Source: three-view drawing plus pictorial views. Frame: mm from the lowest corner of the part. A direction names the side the tool comes from. Give positions to 0.01 mm unless a question says otherwise; leave off trailing zeros. Loops run counter-clockwise (first coordinate to the right, second up) from the corner with the lowest first, then second, coordinate; pieces in that order, holes last. Notation, with made-up numbers: (47, -34.75) -> (102, -34.75) arc R15 cw to (102, -17.75) -> close; hole circle Ø1 at (37.25, 72.25). An arc over 180 degrees is marked (long way). Put each result on its own line as item: value.
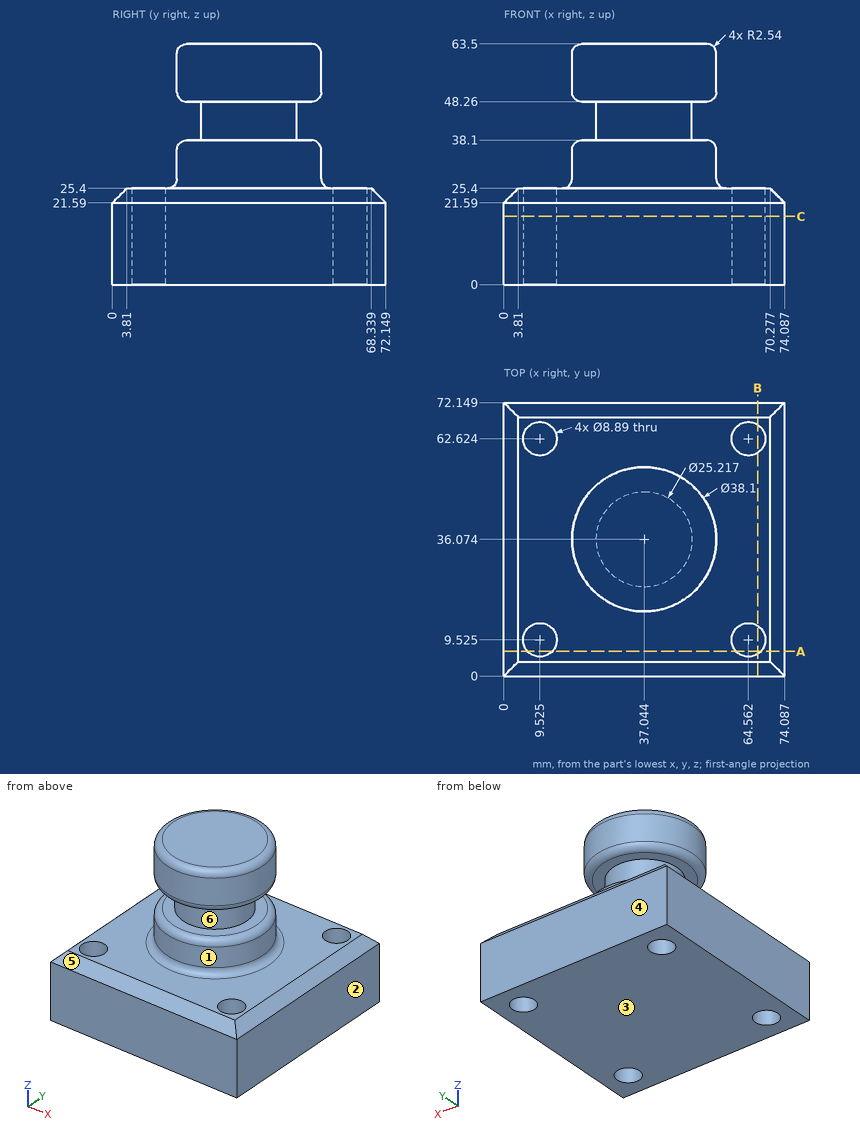
(1) First-contact query: P1, Ø4, axis at x = 31.5, z = 57, coming from the +Y side; P2, Ø12, axis at y = 16, z = 29, coming from the -X side; P3, Ø12, axis at x = 58.5, y = 14, coming from the +Z side. Flat tips, straight axial feed; report the tip coordinate or a pass-through.
Calculated:
P1: stops at y = 54.79
P2: stops at x = 1.41
P3: stops at z = 25.4
(2) Section A-A on y = 6.5. Return loops of the section in (x, z) (1 decimal).
Calculated:
outline: (0, 0) -> (6.3, 0) -> (6.3, 25.4) -> (3.8, 25.4) -> (0, 21.6) -> close; (12.8, 0) -> (61.3, 0) -> (61.3, 25.4) -> (12.8, 25.4) -> close; (67.8, 0) -> (74.1, 0) -> (74.1, 21.6) -> (70.3, 25.4) -> (67.8, 25.4) -> close
(3) Line query: probe 1 along Y at (x, z) = (10.5, 6); probe 2 along Z at (x, y) = (13, 4); probe 3 along Y at (x, z) = (9, 15). Output: solid intervals per line, ascending. Write a range as from..to.
Calculated:
probe 1: y = 0..5.19, 13.86..58.29, 66.96..72.15
probe 2: z = 0..25.4
probe 3: y = 0..5.11, 13.94..58.21, 67.04..72.15
(4) Section C-C on z = 18. Return loops of the section in (x, y) (1 decimal).
Calculated:
outline: (0, 0) -> (74.1, 0) -> (74.1, 72.1) -> (0, 72.1) -> close; hole circle Ø8.9 at (9.5, 9.5); hole circle Ø8.9 at (9.5, 62.6); hole circle Ø8.9 at (64.6, 9.5); hole circle Ø8.9 at (64.6, 62.6)
(5) Reachability of the marked faces 1 and 2 from +Z, -Z, +X, -X, +Y, -Y: full face, straight path, thin tool, end or side. Return the list, or none.
Calculated:
face 1: +Z
face 2: +Z, -Z, +X, +Y, -Y
(6) Section B-B on x = 67. Return loops of the section in (y, z).
Calculated:
outline: (0, 0) -> (5.81, 0) -> (5.81, 25.4) -> (3.81, 25.4) -> (0, 21.59) -> close; (13.24, 0) -> (58.91, 0) -> (58.91, 25.4) -> (13.24, 25.4) -> close; (66.34, 0) -> (72.15, 0) -> (72.15, 21.59) -> (68.34, 25.4) -> (66.34, 25.4) -> close
(7) Draft query along Z for the marked faces 3, 4, 5 and 6. Return one class per face: released by +Z, released by -Z, zero draft, split by the parting line, or undercut.
Calculated:
face 3: released by -Z
face 4: zero draft
face 5: released by +Z
face 6: undercut
